Verification items for this drawing (mm, ordinates from the low corner). Coordinates: 2 decimals unless noted, no trailing zeros. Write each loop counter-clockwise with the first axis right and the second up, starting at its lowest first coordinate (ties: lowest second). Pieces come first, ordered by that corner, then holes. Notation, with made-up numbers: M 4,44.5 L 34,44.5 A22 ccw 34,63.5 Z; hole C 44.25,-4.5 d9. An arc over 180 degrees is marked long. Put each result on its own line as item: value. Start each with the question number.
1) Cross-section at A-A on y = 12.25. Record the cut outline in (x, z).
2) Gauge pin test, flat ends, axial feed: pin 1 (1 mm diameter, centred on x = 4, y = 8, fed in from +Z) (1 decimal); pin 2 (15 mm diameter, centred on x = 17.32, z = 15, fed in from +Y); pin 3 (4 mm diameter, centred on y = 5, z = 12.5, fed in from +X); pin 4 (4 mm diameter, centred on x = 28.5, y = 5, fed in from -Z). Record the tip position at first contact, or that the pin passes through.
3) Mould release check, pull along X, two halves, no side actions. Record for the marked faces 1, 2 and 3: released by +X, released by -X, zero draft, split by the parting line, or undercut.
4) Scan lines: line 1 along X through (y, z) = (10.5, 15); line 2 along Z through (x, y) = (17.5, 5); line 3 along X through (y, z) = (4.75, 11.5). Record each from-to range of solid material in increasing order.
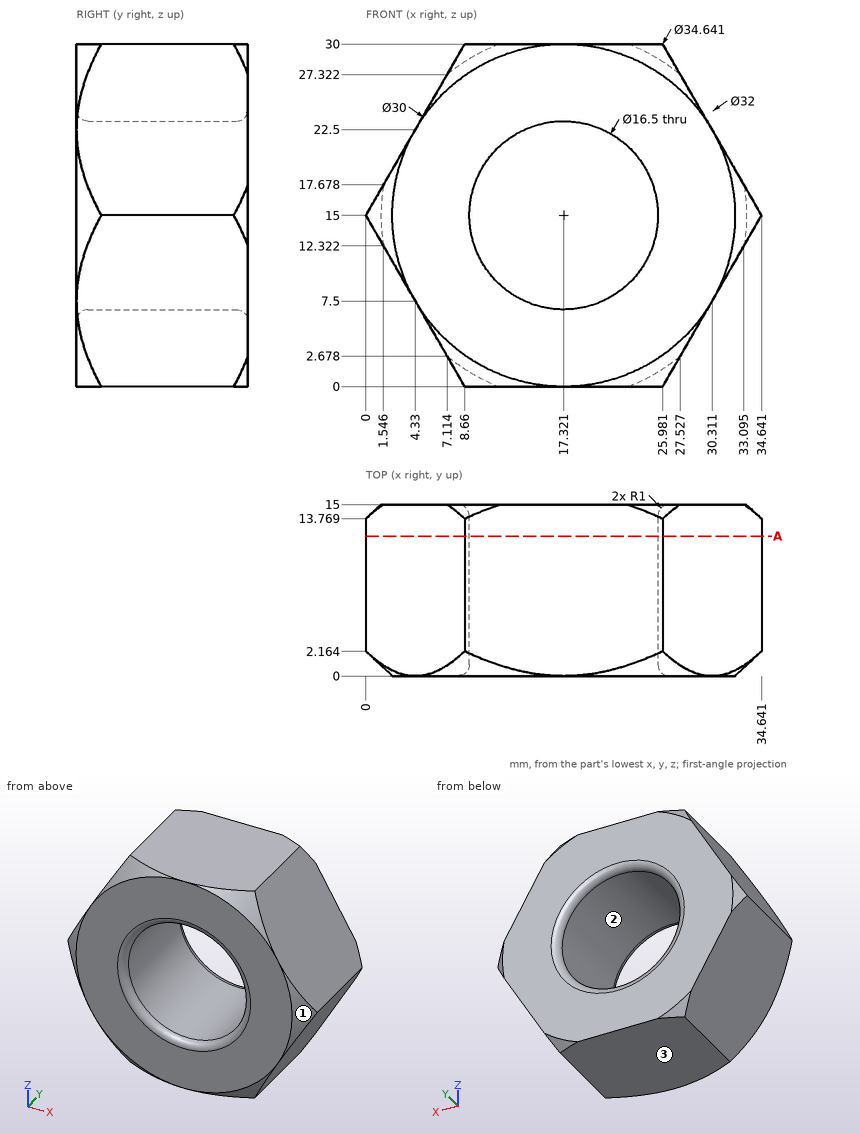
Answer key:
1. outline: M 0,15 L 8.66,0 L 25.98,0 L 34.64,15 L 25.98,30 L 8.66,30 Z; hole C 17.32,15 d16.5
2. pin 1: stops at z = 22.8
2. pin 2: passes through
2. pin 3: stops at x = 34.35
2. pin 4: stops at z = 0.9
3. face 1: released by +X
3. face 2: undercut
3. face 3: zero draft
4. line 1: x = 0 to 9.07, 25.57 to 34.64
4. line 2: z = 0 to 6.75, 23.25 to 30
4. line 3: x = 2.02 to 9.85, 24.79 to 32.62
